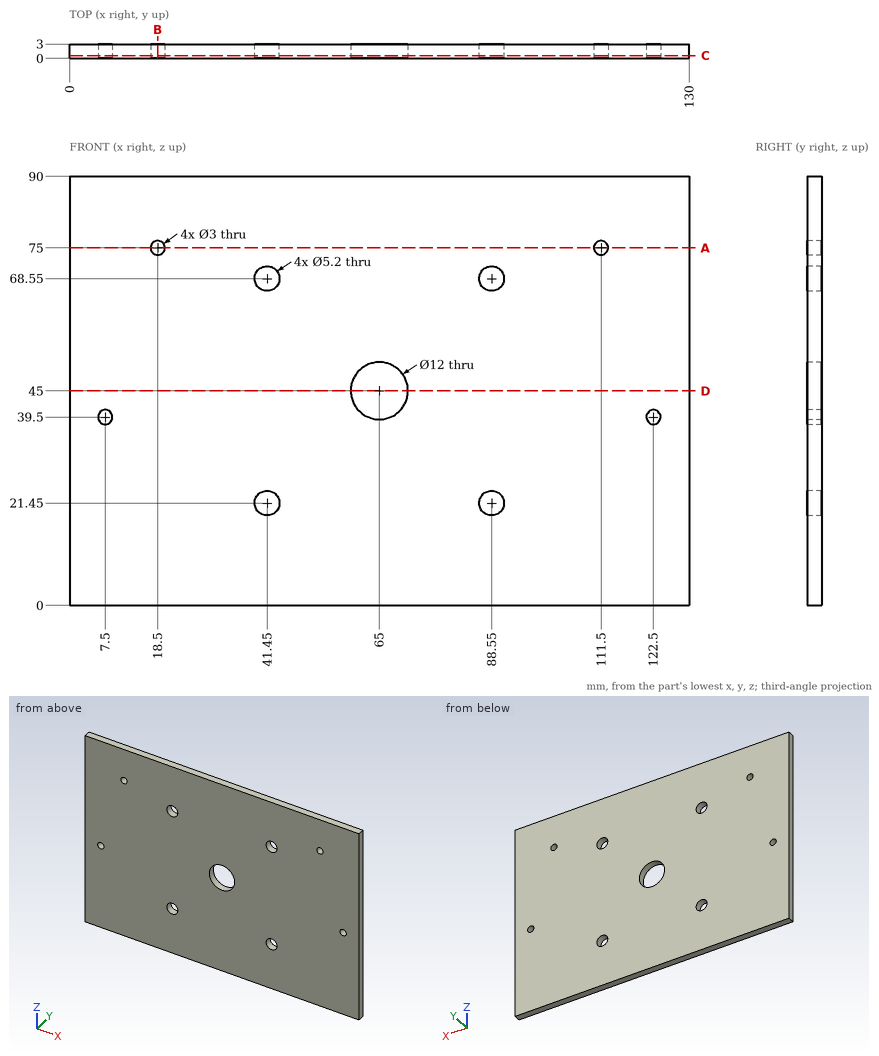
Job drawing, mm, ordinate dimensions from the low corner. One solid piece. Give positions to 0.01 mm unless a question says otherwise; leave off trailing zeros. Loops run counter-clockwise (first coordinate to the right, second up) from the corner with the lowest first, then second, coordinate; pieces in that order, holes last. Notation, with made-up numbers: (42, 17.5) -> (57, 17.5) arc R17 cw to (57, 47.5) -> close; hole circle Ø10 at (33.25, 83). An arc over 180 degrees is marked (long way). Use a Markdown table: item, result. Add a question column.
(1) Wall check: line 1 along X through (y, z) = (2.1, 68.55); line 2 along X through (y, z) = (1.7, 75); line 3 along Z through (x, y) = (122.5, 2.2). Give the ranges that are in metal, low to high.
(2) Slice it at B-B on x = 18.5. List the corners of the cut face in (y, z), and give its area (3 significant figures).
(3) Slice it at C-C on y = 0.55. Give the number of separate pieces and of enclosed holes in the cut face, and give its area (3 significant figures).
(4) Slice it at D-D on z = 45. List the corners of the cut face in (x, y).
(5) Slice it at A-A on z = 75. List the corners of the cut face in (x, y), and give its area (3 significant figures).
Filled sheet:
| question | item | result |
|---|---|---|
| 1 | line 1 | 0 to 38.85, 44.05 to 85.95, 91.15 to 130 |
| 1 | line 2 | 0 to 17, 20 to 110, 113 to 130 |
| 1 | line 3 | 0 to 38, 41 to 90 |
| 2 | outline | (0, 0) -> (3, 0) -> (3, 73.5) -> (0, 73.5) -> close; (0, 76.5) -> (3, 76.5) -> (3, 90) -> (0, 90) -> close |
| 2 | area | 261 mm2 |
| 3 | separate pieces | 1 |
| 3 | enclosed holes | 9 |
| 3 | area | 11,500 mm2 |
| 4 | outline | (0, 0) -> (59, 0) -> (59, 3) -> (0, 3) -> close; (71, 0) -> (130, 0) -> (130, 3) -> (71, 3) -> close |
| 5 | outline | (0, 0) -> (17, 0) -> (17, 3) -> (0, 3) -> close; (20, 0) -> (110, 0) -> (110, 3) -> (20, 3) -> close; (113, 0) -> (130, 0) -> (130, 3) -> (113, 3) -> close |
| 5 | area | 372 mm2 |
